```python
from build123d import *


# Not quite as in the source:
# - ends of sketch curves that miss each other by under 0.0002 mm in the source are joined


with BuildPart() as f1:
    # F0 (on Front) → F1 (revolve)
    with BuildSketch(Plane.XZ):
        with BuildLine():
            Line((4, 21), (18.25, 21))
            Line((18.25, 21), (18.5, 21.25))
            Line((18.5, 21.25), (18.75, 21))
            Line((18.75, 21), (33, 21))
            ThreePointArc((33, 21), (35.8284271247, 22.1715728753), (37, 25))
            Line((37, 25), (37, 27.5))
            Line((37, 27.5), (36.4, 27.5))
            Line((36.4, 27.5), (36.4, 27))
            Line((36.4, 27), (35.4, 27))
            Line((35.4, 27), (35.4, 28))
            Line((35.4, 28), (32.214393, 28))
            ThreePointArc((32.214393, 28), (30.1823197382, 25.3531604535), (26.99975, 24.35))
            Line((26.99975, 24.35), (18.75, 24.35))
            Line((18.75, 24.35), (18.5, 24.1))
            Line((18.5, 24.1), (18.25, 24.35))
            Line((18.25, 24.35), (17.5, 24.35))
            Line((17.5, 24.35), (17.5, 23.25))
            Line((17.5, 23.25), (15.5, 23.25))
            Line((15.5, 23.25), (15.5, 24.35))
            Line((15.5, 24.35), (10.00025, 24.35))
            ThreePointArc((10.00025, 24.35), (6.9048905694, 25.3595695979), (5.0000000057, 28.0000000018))
            Line((5.0000000057, 28.0000000018), (1.6, 28))
            Line((1.6, 28), (1.6, 27))
            Line((1.6, 27), (0.6, 27))
            Line((0.6, 27), (0.6, 27.5))
            Line((0.6, 27.5), (0, 27.5))
            Line((0, 27.5), (0, 25))
            ThreePointArc((0, 25), (1.1715728753, 22.1715728753), (4, 21))
        make_face()
    revolve(axis=Axis((18.5, 0, 0), (1, 0, 0)))


solid = f1.part
```
The listing builds one solid part. Answer for the finished solid, in the listing's coordinates (mm). A direction names the side the tool comes from. Round coordinates to 2 decimals unless told otherwise and drop trailing zeros. Write each loop counter-clockwise with the first axis right and the second up, starting at its lowest first coordinate (ties: lowest second). Pieces come first, ordered by that corner, then holes. Notation, with made-up numbers: (82.25, -15) -> (120.25, -15) arc R32 ccw to (120.25, 16) -> close; hole circle Ø6 at (29, -24.75). An arc over 180 degrees is marked (long way). Use CSV: the item, a comma, the result in double quotes. Start each with the question number.
(1) Consider L1, parallel to Z at x = 26.5, y = 0; L2, parallel to X at y = -24.5, z = -13. Determine where each line is inside the solid, lowest interval first. Write a range as from..to.
(2) Each of these flat-tipped pins is pushed along its axis until it touches: pin 1 (3 mm diameter, centred on x = 24, z = 21.5, fed in from +Y); pin 2 (2 mm diameter, centred on x = 27.5, y = 3.5, fed in from -Z); pin 3 (10 mm diameter, centred on x = 17, y = 2, fed in from +Z). Where does it stop, or does it pass through?
(3) The mould has two halves that part along Z. Classify faces 1 (the face through (22.82, 14.82, -19.32)), 2 (the face through (11.22, -6.31, 20.03)), 3 (the face through (0.6, 18.2, -20.2)), 4 (the face through (25.97, -6.31, 20.03)): released by +Z, released by -Z, zero draft, split by the parting line, or undercut.
(4) Which of the six approach directions +Z, -Z, +X, -X, +Y, -Y give full straight-line access (tool end or side, diameter ignored) to faces 5 (the face through (17.87, 14.82, -19.32)), 6 (the face through (33.785, 10.724, 25.865)), 7 (the face through (36.696, 26.846, -5.961))?
(5) Section A-A on x = 6.5 is taken. Give the vertices of the cut face in (y, z).
(6) Section B-B on x = 30 is taken. Give the vertices of the cut face in (y, z).
A:
1,L1,"z = -24.35..-21, 21..24.35"
1,L2,"x = 1.6..5.09, 32.11..35.4"
2,pin 1,"stops at y = 13.89"
2,pin 2,"stops at z = -24.34"
2,pin 3,"stops at z = 24.35"
3,face 1,"split by the parting line"
3,face 2,"undercut"
3,face 3,"zero draft"
3,face 4,"undercut"
4,face 5,"none"
4,face 6,"+X, -X"
4,face 7,"+X"
5,outline,"circle Ø51.37 at (0, 0); hole circle Ø42 at (0, 0)"
6,outline,"circle Ø50.46 at (0, 0); hole circle Ø42 at (0, 0)"
